Can you work these out from the model? Positions are in its coordinate system, mm. Face numbers are marked on the shaded views. A direction names the side the tool comes from. Coordinates: 2 decimals unless noted, no trailing zeros. Loops run counter-clockwise (first coordinate to the right, second up) from the corner with the lowest first, then second, coordinate; pieces in that order, holes last. Notation, with made-up numbers: (70.5, 78) -> (103.5, 78) arc R5 ccw to (103.5, 86) -> close; hole circle Ø7 at (-3, 77.5). An arc over 180 degrees is marked (long way). Use one line per item in the form item = value. Start each with the question number.
(1) I need wall thicknesses on line 1 (X direction, y = 33, z = -40); line 2 (Z direction, x = -25.5, y = 23.5) (3 decimals); line 3 (X direction, y = 40.5, z = 71). Which ranges of each line are inside material? Lowest first, please. Write a range as [from, to].
(2) Imagine slicing it at D-D (z = -34). List the corners of the cut face in (x, y) for me (3 decimals).
(3) On a 3-axis mill with a long thin cutter (end or side, diameter ignored), from which of +Z, -Z, +X, -X, +Y, -Y can I reach the whole of each face in a straight line? I mean the marked faces 4 and 5. Say none if no direction works.
(4) Imagine slicing it at C-C (y = 3). List the corners of the cut face in (x, z) for me (3 decimals), plus the area to 3 significant figures.
(5) Imagine slicing it at B-B (x = 20). List the corners of the cut face in (y, z) for me (3 decimals).
(6) Imagine slicing it at A-A (y = 41). List the corners of the cut face in (x, z) for me (3 decimals).
(7) Thinking about a two-plate mould opening in X: for the marked faces 1, 2 and 3, which applies, released by +X, released by -X, zero draft, split by the parting line, or undercut?
(8) I'm going to push flat-ended pins straight in: pin 1 (7.5 mm diameter, centred on y = 29.5, z = -33, fed in from +X); pin 2 (2.5 mm diameter, centred on x = -1.5, y = 2.5, fed in from +Z); pin 3 (5 mm diameter, centred on x = 11, z = 16, fed in from +Y); pin 4 (1.5 mm diameter, centred on y = 3, z = 2.5, fed in from +X). Where does each tip first touch, or does it pass through?
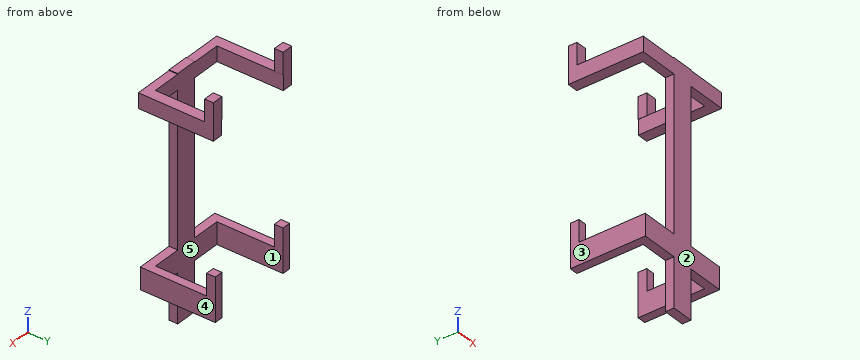
Autodesk Inventor part; units mm, degrees
ref_plane "YZ Plane" through (0, 0, 0) normal (1, 0, 0) x (0, 1, 0)
ref_plane "XZ Plane" through (0, 0, 0) normal (0, 1, 0) x (-1, 0, 0)
ref_plane "XY Plane" through (0, 0, 0) normal (0, 0, 1) x (1, 0, 0)
sketch "Sketch1" plane through (0, 0, 0) normal (0, 1, 0) x (-1, 0, 0)
  line L0 (23.114, 69.469) -> (-23.114, 69.469)
  line L1 (-23.114, 69.469) -> (-23.114, -69.469)
  line L2 (-23.114, -69.469) -> (23.114, -69.469)
  line L3 (23.114, -69.469) -> (23.114, 69.469)
  line L4 (23.114, 69.469) -> (-23.114, -69.469) construction
  line L5 (-23.114, 69.469) -> (23.114, -69.469) construction
  line L6 (-29.464, 60.706) -> (29.464, 60.706)
  line L7 (29.464, 60.706) -> (29.464, 69.469)
  line L8 (29.464, 69.469) -> (-29.464, 69.469)
  line L9 (-29.464, 69.469) -> (-29.464, 60.706)
  line L10 (-29.464, 60.706) -> (29.464, 69.469) construction
  line L11 (29.464, 60.706) -> (-29.464, 69.469) construction
  line L12 (6.35, 69.85) -> (-6.35, 69.85)
  line L13 (-6.35, 69.85) -> (-6.35, -69.85)
  line L14 (-6.35, -69.85) -> (6.35, -69.85)
  line L15 (6.35, -69.85) -> (6.35, 69.85)
  line L16 (6.35, 69.85) -> (-6.35, -69.85) construction
  line L17 (-6.35, 69.85) -> (6.35, -69.85) construction
  point P0 (0, 0)
  point P1 (0, 65.0875)
  dimension "d0" = 46.228
  dimension "d1" = 138.938
  dimension "d2" = 58.928
sketch "Sketch2" plane through (0, 0, 0) normal (0, 1, 0) x (-1, 0, 0)
  line L0 (-9.525, 69.85) -> (-9.525, -28.575)
  line L1 (-38.1, -41.275) -> (38.1, -41.275)
  line L2 (38.1, -41.275) -> (38.1, -28.575)
  line L3 (38.1, -28.575) -> (-38.1, -28.575)
  line L4 (-38.1, -28.575) -> (-38.1, -41.275)
  line L5 (-38.1, -41.275) -> (38.1, -28.575) construction
  line L6 (38.1, -41.275) -> (-38.1, -28.575) construction
  point P0 (0, 0)
  point P1 (0, -34.925)
  dimension "d3" = 98.425
  dimension "d4" = 76.2
extrude "Extrusion1" add sketch "Sketch2" along normal blind 5.08
extrude "Extrusion2" add sketch "Sketch1" along normal blind 5.08 contours L3 L6 L15 L0 | L8 L7 L6 L3 | L15 L6 L13 L0 | L0 L13 L12 L15 | L13 L6 L1 L0 | L15 L2 L13 L6 | L1 L6 L9 L8 | L15 L14 L13 L2
sketch "Sketch3" plane through (0, 5.08, 0) normal (0, 1, 0) x (1, 0, 0)
  line L0 (-29.464, -60.706) -> (-29.464, -69.469)
  line L1 (-29.464, -69.469) -> (-6.35, -69.469)
  line L2 (-29.464, -60.706) -> (-23.114, -60.706)
  line L3 (-23.114, -60.706) -> (-23.114, -69.469)
  line L4 (-23.114, -69.469) -> (-29.464, -69.469)
  line L5 (-29.464, -69.469) -> (-29.464, -60.706)
  line L6 (29.464, -69.469) -> (29.464, -60.706)
  line L7 (6.35, -69.469) -> (29.464, -69.469)
  line L8 (29.464, -60.706) -> (23.114, -60.706)
  line L9 (23.114, -60.706) -> (23.114, -69.469)
  line L10 (23.114, -69.469) -> (29.464, -69.469)
  line L11 (29.464, -69.469) -> (29.464, -60.706)
  point P0 (0, 0)
  dimension "d9" = 6.35
  dimension "d10" = 6.35
extrude "Extrusion3" add sketch "Sketch3" along normal blind 38.735
sketch "Sketch4" plane through (0, 5.08, 0) normal (0, 1, 0) x (1, 0, 0)
  line L0 (-38.1, 41.275) -> (-38.1, 28.575)
  line L1 (-38.1, 28.575) -> (-6.35, 28.575)
  line L2 (-38.1, 41.275) -> (-22.987, 41.275)
  line L3 (-22.987, 41.275) -> (-22.987, 28.575)
  line L4 (-22.987, 28.575) -> (-38.1, 28.575)
  line L5 (-38.1, 28.575) -> (-38.1, 41.275)
  line L6 (38.1, 28.575) -> (38.1, 41.275)
  line L7 (6.35, 28.575) -> (38.1, 28.575)
  line L8 (38.1, 41.275) -> (22.987, 41.275)
  line L9 (22.987, 41.275) -> (22.987, 28.575)
  line L10 (22.987, 28.575) -> (38.1, 28.575)
  line L11 (38.1, 28.575) -> (38.1, 41.275)
  point P0 (0, 0)
  dimension "d13" = 15.113
  dimension "d14" = 15.113
extrude "Extrusion4" add sketch "Sketch4" along normal blind 38.735
sketch "Sketch5" plane through (-38.1, 0, -41.275) normal (-1, 0, 0) x (0, 0, 1)
  line L0 (-6.35, 53.975) -> (19.05, 53.975)
  line L1 (19.05, 53.975) -> (19.05, -3.175)
  line L2 (19.05, -3.175) -> (-6.35, -3.175)
  line L3 (-6.35, -3.175) -> (-6.35, 53.975)
  line L4 (-6.35, 53.975) -> (19.05, -3.175) construction
  line L5 (19.05, 53.975) -> (-6.35, -3.175) construction
  point P0 (41.275, 0)
  point P1 (6.35, 25.4)
extrude "Extrusion5" cut sketch "Sketch5" against normal blind 10.16
sketch "Sketch6" plane through (6.35, 0, -28.575) normal (0, 0, 1) x (1, 0, 0)
  point P0 (-6.35, 0)
sketch "Sketch7" plane through (38.1, 0, -28.575) normal (1, 0, 0) x (0, 0, -1)
  line L0 (-1.5875, 49.2125) -> (17.4625, 49.2125)
  line L1 (17.4625, 49.2125) -> (17.4625, -4.7625)
  line L2 (17.4625, -4.7625) -> (-1.5875, -4.7625)
  line L3 (-1.5875, -4.7625) -> (-1.5875, 49.2125)
  line L4 (-1.5875, 49.2125) -> (17.4625, -4.7625) construction
  line L5 (17.4625, 49.2125) -> (-1.5875, -4.7625) construction
  point P0 (-28.575, 0)
  point P1 (7.9375, 22.225)
extrude "Extrusion6" cut sketch "Sketch7" against normal blind 10.16
sketch "Sketch8" plane through (-29.464, 0, 69.469) normal (0, 0, 1) x (1, 0, 0)
  line L0 (0, 0) -> (0, 43.815)
  line L1 (6.477, 5.08) -> (6.477, 43.815)
  line L2 (0, 43.815) -> (6.477, 43.815)
  line L3 (6.477, 43.815) -> (6.477, 38.735)
  line L4 (6.477, 38.735) -> (0, 38.735)
  line L5 (0, 38.735) -> (0, 43.815)
  line L6 (58.928, 0) -> (58.928, 43.815)
  line L7 (52.451, 5.08) -> (52.451, 43.815)
  line L8 (58.928, 43.815) -> (52.451, 43.815)
  line L9 (52.451, 43.815) -> (52.451, 38.735)
  line L10 (52.451, 38.735) -> (58.928, 38.735)
  line L11 (58.928, 38.735) -> (58.928, 43.815)
  point P0 (29.464, 0)
  dimension "d21" = 5.08
extrude "Extrusion7" add sketch "Sketch8" along normal blind 12.7
sketch "Sketch9" plane through (6.35, 0, -28.575) normal (0, 0, 1) x (1, 0, 0)
  line L0 (16.637, 5.08) -> (16.637, 43.815)
  line L1 (21.59, 43.815) -> (21.59, 0)
  line L2 (16.637, 43.815) -> (21.59, 43.815)
  line L3 (21.59, 43.815) -> (21.59, 38.735)
  line L4 (21.59, 38.735) -> (16.637, 38.735)
  line L5 (16.637, 38.735) -> (16.637, 43.815)
  line L6 (-34.29, 43.815) -> (-34.29, 0)
  line L7 (-29.337, 5.08) -> (-29.337, 43.815)
  line L8 (-34.29, 43.815) -> (-29.337, 43.815)
  line L9 (-29.337, 43.815) -> (-29.337, 38.735)
  line L10 (-29.337, 38.735) -> (-34.29, 38.735)
  line L11 (-34.29, 38.735) -> (-34.29, 43.815)
  point P0 (-6.35, 0)
  dimension "d24" = 5.08
extrude "Extrusion8" add sketch "Sketch9" along normal blind 12.7
properties part number "battery"
Worked out:
q1.line_1 = [-27.94, -22.99], [22.99, 27.94]
q1.line_2 = [-41.275, -28.575], [60.706, 69.469]
q1.line_3 = [-29.46, -22.99], [22.99, 29.46]
q2.outline = (-27.94, 0) -> (27.94, 0) -> (27.94, 43.815) -> (22.987, 43.815) -> (22.987, 5.08) -> (-22.987, 5.08) -> (-22.987, 43.815) -> (-27.94, 43.815) -> close
q3.face_4 = -Z, +X, +Y, -Y
q3.face_5 = +Z, -Z, +Y
q4.outline = (-29.464, 60.706) -> (-6.35, 60.706) -> (-6.35, -28.575) -> (-27.94, -28.575) -> (-27.94, -41.275) -> (-6.35, -41.275) -> (-6.35, -69.85) -> (6.35, -69.85) -> (6.35, -41.275) -> (27.94, -41.275) -> (27.94, -28.575) -> (6.35, -28.575) -> (6.35, 60.706) -> (29.464, 60.706) -> (29.464, 69.469) -> (6.35, 69.469) -> (6.35, 69.85) -> (-6.35, 69.85) -> (-6.35, 69.469) -> (-29.464, 69.469) -> close
q4.area = 2,730 mm2
q5.outline = (0, -41.275) -> (5.08, -41.275) -> (5.08, -28.575) -> (0, -28.575) -> close; (0, 60.706) -> (5.08, 60.706) -> (5.08, 69.469) -> (0, 69.469) -> close
q6.outline = (-29.464, 60.706) -> (-23.114, 60.706) -> (-23.114, 69.469) -> (-22.987, 69.469) -> (-22.987, 82.169) -> (-29.464, 82.169) -> close; (-27.94, -41.275) -> (-22.987, -41.275) -> (-22.987, -15.875) -> (-27.94, -15.875) -> close; (22.987, -41.275) -> (27.94, -41.275) -> (27.94, -15.875) -> (22.987, -15.875) -> close; (22.987, 69.469) -> (23.114, 69.469) -> (23.114, 60.706) -> (29.464, 60.706) -> (29.464, 82.169) -> (22.987, 82.169) -> close
q7.face_1 = undercut
q7.face_2 = zero draft
q7.face_3 = released by -X
q8.pin_1 = 27.94
q8.pin_2 = 69.85
q8.pin_3 = through
q8.pin_4 = 6.35
